Verification items for this drawing (mm, ordinates from the low corner). A direction names the side the tool comes from. Round coordinates to 2 decimals unless told otherwise and drop trailing zeros. Loops run counter-clockwise (first coordinate to the right, second up) from the corner with the lowest first, then second, coordinate; pieces in that order, holes last. Notation, with made-up numbers: (62, 34.5) -> (113, 34.5) arc R19 ccw to (113, 67.5) -> close; hole circle Ø9 at (-15, 69). An arc over 180 degrees is marked (long way). One line per question, with ' | ' between items.
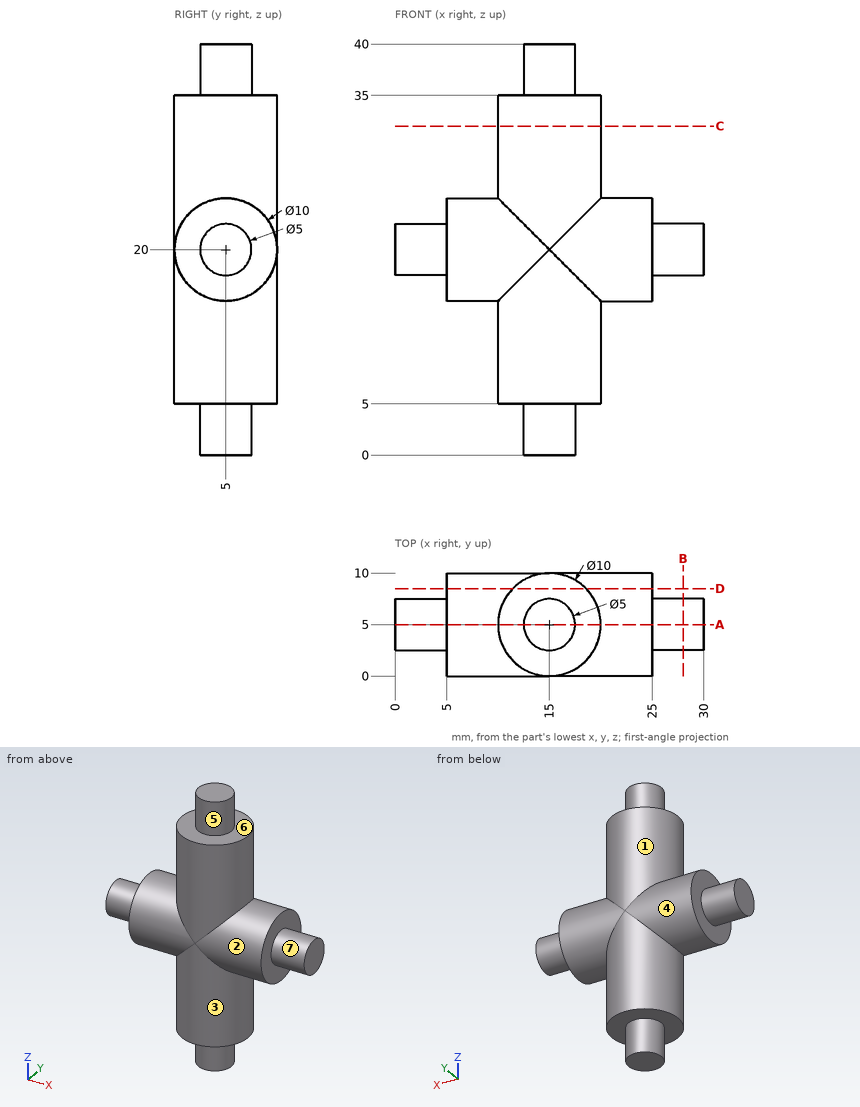
(1) Set-up check for the marked faces 1, 2, 3 and 4: record each of +Z, -Z, +X, -X, +Y, -Y from which the full face is reachable in a straight line by a thin tool's end or side.
Answer:
face 1: +Z | face 2: +X | face 3: -Z | face 4: -X
(2) Mould release check, pull along Z, two halves, no side actions. Record for the marked faces 5, 6 and 7: +Z half, -Z half, draft (parallel to the pull), parting line (faces both ways), or undercut.
Answer:
face 5: draft | face 6: +Z half | face 7: parting line
(3) Scan lines: probe 1 along X at (y, z) = (7, 17); probe 2 along Z at (x, y) = (11.25, 7.5); probe 3 along Y at (x, z) = (13.25, 34.5). Record each from-to range of solid material in increasing order.
Answer:
probe 1: x = 5 to 25 | probe 2: z = 5 to 35 | probe 3: y = 0.32 to 9.68
(4) Sectioned sample at D-D, the plane y = 8.5. Record the cut outline in (x, z), and give its area (3 significant figures).
Answer:
outline: (5, 16.43) -> (11.43, 16.43) -> (11.43, 5) -> (18.57, 5) -> (18.57, 16.43) -> (25, 16.43) -> (25, 23.57) -> (18.57, 23.57) -> (18.57, 35) -> (11.43, 35) -> (11.43, 23.57) -> (5, 23.57) -> close | area: 306 mm2
(5) Sectioned sample at C-C, the plane z = 32. Record the cut outline in (x, y).
Answer:
outline: circle Ø10 at (15, 5)
(6) Sectioned sample at B-B, the plane x = 28. Record the cut outline in (y, z).
Answer:
outline: circle Ø5 at (5, 20)
(7) Go/stop test with flat-tipped pins: pin 1 (1 mm diameter, centred on y = 6.5, z = 23.5, fed in from +X); pin 2 (3 mm diameter, centred on y = 6, z = 21, fed in from -X); pin 3 (2 mm diameter, centred on y = 4.5, z = 33, fed in from +X); pin 4 (1.5 mm diameter, centred on x = 3.5, z = 20.5, fed in from -Y). Record where each tip stops, or that it passes through.
Answer:
pin 1: stops at x = 25 | pin 2: stops at x = 0 | pin 3: stops at x = 20 | pin 4: stops at y = 2.5
(8) Sectioned sample at A-A, the plane y = 5. Record the cut outline in (x, z), and give its area (3 significant figures).
Answer:
outline: (0, 17.5) -> (5, 17.5) -> (5, 15) -> (10, 15) -> (10, 5) -> (12.5, 5) -> (12.5, 0) -> (17.5, 0) -> (17.5, 5) -> (20, 5) -> (20, 15) -> (25, 15) -> (25, 17.5) -> (30, 17.5) -> (30, 22.5) -> (25, 22.5) -> (25, 25) -> (20, 25) -> (20, 35) -> (17.5, 35) -> (17.5, 40) -> (12.5, 40) -> (12.5, 35) -> (10, 35) -> (10, 25) -> (5, 25) -> (5, 22.5) -> (0, 22.5) -> close | area: 500 mm2
